Work out the finished part from the listing and answer in its coordinate system (mm). A direction names the side the tool comes from. Round coordinates to 2 decimals unless told otherwise and drop trailing zeros. Order: outer loops, then holes, each group sorted by start corner. A loop starts at its lowest first (then second) coordinate and runs counter-clockwise, first axis right, second up. Notation, with made-up numbers: (83.25, -15) -> (128.25, -15) arc R11 ccw to (128.25, -5) -> close; hole circle Ø3 at (11, -21.75). An arc over 180 degrees is marked (long way). Use one line per item in the form item = value.
Autodesk Inventor part; units mm, degrees
ref_plane "YZ Plane" through (0, 0, 0) normal (1, 0, 0) x (0, 1, 0)
ref_plane "XZ Plane" through (0, 0, 0) normal (0, 1, 0) x (-1, 0, 0)
ref_plane "XY Plane" through (0, 0, 0) normal (0, 0, 1) x (1, 0, 0)
sketch "Sketch1" plane through (0, 0, 0) normal (0, 0, 1) x (1, 0, 0)
  line L0 (-32.5, 32.5) -> (32.5, 32.5)
  line L1 (32.5, 32.5) -> (32.5, -32.5)
  line L2 (32.5, -32.5) -> (-32.5, -32.5)
  line L3 (-32.5, -32.5) -> (-32.5, 32.5)
  line L4 (-32.5, 32.5) -> (32.5, -32.5) construction
  line L5 (32.5, 32.5) -> (-32.5, -32.5) construction
  point P0 (0, 0)
  dimension "d0" = 65
  dimension "d1" = 65
extrude "Extrusion1" add sketch "Sketch1" along normal blind 3
fillet "Fillet1" radius 8 4 edges at (-32.5, -32.5, 1.5) (32.5, -32.5, 1.5) (32.5, 32.5, 1.5) (-32.5, 32.5, 1.5)
sketch "Sketch2" plane through (0, 0, 0) normal (0, 0, -1) x (-1, 0, 0)
  circle A0 centre (0, 0) radius 15
  dimension "d5" = 30
extrude "Extrusion2" add sketch "Sketch2" along normal blind 10
fillet "Fillet2" radius 3 1 edges at (15, 0, 0)
fillet "Fillet3" radius 1.5 1 edges at (15, 0, -10)
sketch "Sketch3" plane through (0, 0, 3) normal (0, 0, 1) x (1, 0, 0)
  line L0 (-25.5, 25.5) -> (25.5, 25.5)
  line L1 (25.5, 25.5) -> (25.5, -25.5)
  line L2 (25.5, -25.5) -> (-25.5, -25.5)
  line L3 (-25.5, -25.5) -> (-25.5, 25.5)
  line L4 (-25.5, 25.5) -> (25.5, -25.5) construction
  line L5 (25.5, 25.5) -> (-25.5, -25.5) construction
  point P0 (0, 0)
  dimension "d10" = 51
  dimension "d11" = 51
extrude "Extrusion3" cut sketch "Sketch3" against normal blind 1
properties part number "square_with_fillet_65mm"
Item 1: The part is cut by section B-B, the plane x = 0. Give the vertices of the cut face in (y, z).
Findings:
outline = (-32.5, 0) -> (-18, 0) arc R3 cw to (-15, -3) -> (-15, -8.5) arc R1.5 ccw to (-13.5, -10) -> (13.5, -10) arc R1.5 ccw to (15, -8.5) -> (15, -3) arc R3 cw to (18, 0) -> (32.5, 0) -> (32.5, 3) -> (25.5, 3) -> (25.5, 2) -> (-25.5, 2) -> (-25.5, 3) -> (-32.5, 3) -> close
Item 2: Determine the mould class of faces 1 (the flat face through (0, -32.5, 1)), 2 (the flat face through (0, 0, 2)), 3 (the cylindrical face through (-30.094, 30.219, 1.521)) for opening direction Y: released by +Y, released by -Y, zero draft, split by the parting line, or undercut.
Findings:
face_1 = released by -Y
face_2 = undercut
face_3 = released by +Y
Item 3: For faces 4 (the cylindrical face through (14.985, -0.66, -5.712)), 5 (the cylindrical face through (-30.219, -30.094, 1.521)), determine the directions among +Z, -Z, +X, -X, +Y, -Y from which every point of the face is accessible in a straight line to the end or side of a thin tool.
Findings:
face_4 = -Z
face_5 = +Z, -Z, -X, -Y
Item 4: Flat-ended cylindrical pins translate along their axes: P1, Ø4, axis at x = -3.5, y = -2.5, coming from the +Z side; P2, Ø6, axis at y = 1, z = -4, coming from the -X side; P3, Ø4, axis at x = -21, z = -2.5, coming from the -Y side; P4, Ø2, axis at x = -14.5, z = -2, coming from the +Y side. Find the tip coordinate at first contact, or state that the pin passes through.
Findings:
P1 = 2
P2 = -15.74
P3 = through
P4 = 7.17
Item 5: The part is cut by section A-A, the plane y = 20.5. Give the vertices of the cut face in (x, z), and give its area (3 significant figures).
Findings:
outline = (-32.5, 0) -> (32.5, 0) -> (32.5, 3) -> (25.5, 3) -> (25.5, 2) -> (-25.5, 2) -> (-25.5, 3) -> (-32.5, 3) -> close
area = 144 mm^2
Item 6: Consider line 1 along X through (y, z) = (0, 2.25); line 2 along Z through (x, y) = (7.5, 6.5). Determine where each line is inside the solid, lowest interval first.
Findings:
line_1 = -32.5 to -25.5, 25.5 to 32.5
line_2 = -10 to 2
Item 7: The part is cut by section C-C, the plane z = -6.25. Give the vertices of the cut face in (x, y).
Findings:
outline = circle Ø30 at (0, 0)
